Can you work these out from the model? Positions are in its coordinate system, mm. Face numbers are marked on the shaded views. A direction names the side the tool comes from. Coordinates: 2 decimals unless noted, no trailing zeros. Order: outer loops, then holes, each group sorted by start corner. A loop starts at its lowest first (then second) coordinate and runs counter-clockwise, first axis right, second up. Notation, with made-up numbers: (-8.75, 37.5) -> (27.25, 37.5) arc R34 cw to (27.25, 69.5) -> close; hole circle Ø9 at (43, 20). An arc over 180 degrees is marked (long way). Return JSON: item names as keys, results as strings. Group by question number.
1) If we section it at A-A, the plane x = -6.5: Please give me the cut outline in (y, z), then the cut area to 3 significant figures.
2) Thinking about a two-plate mould opening in Z: for the marked faces 3, 4, 5 and 6, which applies, +Z half, -Z half, draft (parallel to the pull), parting line (faces both ways), or undercut?
3) For the marked faces 1 and 2, which set-ups out of +Z, -Z, +X, -X, +Y, -Y let a thin tool reach every point of the face, with its end or its side?
4) If we section it at D-D, the plane y = 161: Please give me the cut outline in (x, z).
5) For pin 1 (8 mm diameter, centred on x = -20.5, z = 20, fed in from -Y); pin 2 (3 mm diameter, centred on x = -14.5, z = 6, fed in from -Y), each with a flat end and sliding along its axis, tell me the tip position at first contact or that it passes through.
6) If I drill on probe 1 along Z at (x, y) = (-19.5, 132); probe 2 along X at (y, z) = (126.5, 4.75); probe 3 along Z at (x, y) = (-12.5, 152), over which ranges is the centre line in solid material (lowest first)? Write a range as from..to.
7) If we section it at B-B, the plane z = 7.75: Please give me the cut outline in (x, y), then the cut area to 4 significant figures.
8) If we section it at C-C, the plane y = 129: Please give me the cut outline in (x, z).
Autodesk Inventor part; units mm, degrees
ref_plane "YZ Plane" through (0, 0, 0) normal (1, 0, 0) x (0, 1, 0)
ref_plane "XZ Plane" through (0, 0, 0) normal (0, 1, 0) x (-1, 0, 0)
ref_plane "XY Plane" through (0, 0, 0) normal (0, 0, 1) x (1, 0, 0)
sketch "Sketch1" plane through (0, 0, 0) normal (0, 1, 0) x (-1, 0, 0)
  line L0 (0, 0) -> (25, 0)
  line L1 (25, 0) -> (25, 25)
  line L2 (25, 25) -> (0, 25)
  line L3 (0, 25) -> (0, 0)
  line L4 (22, 22) -> (22, 3)
  line L5 (22, 3) -> (3, 3)
  line L6 (3, 3) -> (3, 22)
  line L7 (3, 22) -> (22, 22)
  dimension "d0" = 25
  dimension "d1" = 25
  dimension "d2" = 3
extrude "Extrusion1" add sketch "Sketch1" along normal blind 167.25
sketch "Sketch4" plane through (0, 0, 25) normal (1, 0, 0) x (0, 0, -1)
  line L0 (0, 0) -> (25, 0)
  line L1 (25, 0) -> (25, 167.25)
  line L2 (0, 167.25) -> (25, 167.25)
  line L3 (0, 0) -> (0, 167.25)
  line L4 (0, 167.25) -> (25, 142.25)
  line L5 (0, 167.25) -> (35.3553, 167.25) construction
  line L6 (0, 167.25) -> (0, 97.25)
  line L7 (0, 0) -> (0, 167.25)
  line L8 (0, 97.25) -> (25, 97.25)
  line L9 (25, 142.25) -> (25, 97.25)
  dimension "d12" = 45
  dimension "d13" = 70
extrude "Extrusion4" cut sketch "Sketch4" against normal through all contours L3 L8 L1 L0 | L2 L1 L4
properties part number "P602" material "Aluminum 6061"
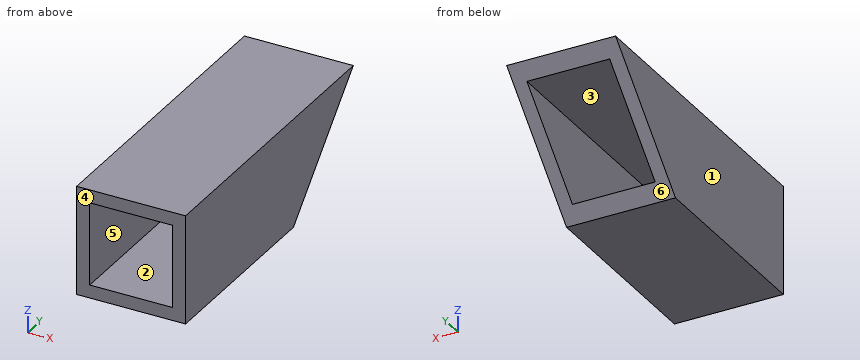
Result sheet:
{
 "1": {"outline": "(97.25, 0) -> (142.25, 0) -> (145.25, 3) -> (97.25, 3) -> close; (97.25, 22) -> (164.25, 22) -> (167.25, 25) -> (97.25, 25) -> close", "area": "345 mm2"},
 "2": {"face 3": "undercut", "face 4": "draft", "face 5": "undercut", "face 6": "-Z half"},
 "3": {"face 1": "+Z, -Z, -X, +Y, -Y", "face 2": "+Y, -Y"},
 "4": {"outline": "(-25, 18.75) -> (-22, 18.75) -> (-22, 22) -> (-3, 22) -> (-3, 18.75) -> (0, 18.75) -> (0, 25) -> (-25, 25) -> close"},
 "5": {"pin 1": "stops at y = 97.25", "pin 2": "passes through"},
 "6": {"probe 1": "z = 0..3, 22..25", "probe 2": "x = -25..-22, -3..0", "probe 3": "z = 22..25"},
 "7": {"outline": "(-25, 97.25) -> (-22, 97.25) -> (-22, 150) -> (-25, 150) -> close; (-3, 97.25) -> (0, 97.25) -> (0, 150) -> (-3, 150) -> close", "area": "316.5 mm2"},
 "8": {"outline": "(-25, 0) -> (0, 0) -> (0, 25) -> (-25, 25) -> close; hole (-22, 3) -> (-3, 3) -> (-3, 22) -> (-22, 22) -> close"}
}
